from build123d import *

# Parameters (mm, degrees)
SKETCH_1_W          = 40
SKETCH_1_H          = 5
EXTRUDE_1_DEPTH     = 200
SKETCH_2_R          = 16
CUT_EXTRUDE_1_DEPTH = 6
SKETCH_3_W          = 40
SKETCH_3_H          = 10
CUT_EXTRUDE_2_DEPTH = 6


with BuildPart() as part:
    # Эскиз1 → Бобышка-Вытянуть1 (new body)
    with BuildSketch(Plane.XY):
        with Locations((20, -2.5)):
            Rectangle(SKETCH_1_W, SKETCH_1_H)
    extrude(amount=EXTRUDE_1_DEPTH)

    # Эскиз2 → Вырез-Вытянуть1 (cut, through all)
    with BuildSketch(Plane(origin=(0, 0, 0), x_dir=(1, 0, 0), z_dir=(0, 1, 0))):
        with Locations((20, -200)):
            Circle(SKETCH_2_R)
    extrude(amount=-CUT_EXTRUDE_1_DEPTH, mode=Mode.SUBTRACT)

    # Эскиз3 → Вырез-Вытянуть2 (cut, through all)
    with BuildSketch(Plane.XZ.offset(5)):
        with Locations((20, 195)):
            Rectangle(SKETCH_3_W, SKETCH_3_H)
    extrude(amount=-CUT_EXTRUDE_2_DEPTH, mode=Mode.SUBTRACT)


solid = part.part
Work out the finished part from the listing and answer in its coordinate system (mm). Round coordinates to 2 decimals unless told otherwise and drop trailing zeros. Write each loop counter-clockwise with the first axis right and the second up, starting at its lowest first coordinate (ties: lowest second). Pieces come first, ordered by that corner, then holes. Notation, with made-up numbers: (76.5, -8.5) -> (92.5, -8.5) arc R24 cw to (92.5, 18.5) -> close; hole circle Ø9 at (-6.5, 14). An arc over 180 degrees is marked (long way). Answer as CSV lines item,"result". Start each with the question number.
(1) Find the intervals of material crossed by probe 1 along Z at (x, y) = (11, -4.4); probe 2 along Z at (x, y) = (21.5, -0.5), in increasing order.
(2) The mould has two halves that part along X. Classify faces 1 (the cylindrical face through (20, -2, 184)), 2 (the flat face through (20, -5, 94)), 3 (the flat face through (40, -3, 94)), 4 (the flat face through (0, -3, 94)): +X half, -X half, draft (parallel to the pull), parting line (faces both ways), or undercut.
(3) The part is cut by section B-B, the plane x = 27.5. Give the vertices of the cut face in (y, z).
(4) The part is cut by section A-A, the plane x = 11.5. Give the vertices of the cut face in (y, z), then the cut area to 3 significant figures.
Output values:
1,probe 1,"z = 0 to 186.77"
1,probe 2,"z = 0 to 184.07"
2,face 1,"undercut"
2,face 2,"draft"
2,face 3,"+X half"
2,face 4,"-X half"
3,outline,"(-5, 0) -> (0, 0) -> (0, 185.87) -> (-5, 185.87) -> close"
4,outline,"(-5, 0) -> (0, 0) -> (0, 186.44) -> (-5, 186.44) -> close"
4,area,"932 mm²"
